Source: CAD feature listing. Evaluate the final solid. Frame: model axes, mm. A direction names the side the tool comes from. Coordinates: 2 decimals unless noted, no trailing zeros. Write each loop counter-clockwise with the first axis right and the second up, starting at its lowest first coordinate (ties: lowest second). Pieces come first, ordered by that corner, then holes. Notation, with made-up numbers: (34.5, -28) - (60.5, -28) arc R35 cw to (60.5, 11) - close; hole circle Ø9 at (16, 56). An arc over 180 degrees is marked (long way). One line per question, with ' | ' between items.
from build123d import *

# Parameters (mm, degrees)
CUT_EXTRUDE1_DEPTH      = 103.528044944
CUT_EXTRUDE1_DEPTH_BACK = 103.528044944
CUT_EXTRUDE2_DEPTH      = 104.553789555
CUT_EXTRUDE2_DEPTH_BACK = 104.553789555


with BuildPart() as part:
    # Sketch1 → Revolve1 (revolve)
    with BuildSketch(Plane.XY, mode=Mode.PRIVATE) as revolve1_sk:
        Polygon((0, 100), (-16, 10), (-16, 0), (0, 0), align=None)
    revolve(revolve1_sk.sketch.rotate(Axis((0, 0, 0), (0, 1, 0)), 270), axis=Axis((0, 0, 0), (0, 1, 0)))

    # Sketch3 → Cut-Extrude1 (cut, two sides: drawn at the far end of the back side and taken through both)
    with BuildSketch(Plane(origin=(0, 0, 0), x_dir=(0, 0, -1), z_dir=(1, 0, 0)).offset(-CUT_EXTRUDE1_DEPTH_BACK)):
        Polygon((-29.451982923, 10), (-6.451982923, 10), (-2.451982923, 110.819600833), (-29.451982923, 110.819600833), align=None)
        Polygon((29.451982923, 10), (6.451982923, 10), (2.451982923, 110.819600833), (29.451982923, 110.819600833), align=None)
    extrude(amount=CUT_EXTRUDE1_DEPTH + CUT_EXTRUDE1_DEPTH_BACK, mode=Mode.SUBTRACT)

    # Sketch4 → Cut-Extrude2 (cut, two sides: drawn at the far end of the back side and taken through both)
    with BuildSketch(Plane(origin=(0, 0.271295166, 6.837967583), x_dir=(1, 0, 0), z_dir=(0, 0.03964363571474905, 0.9992138820829684)).offset(-CUT_EXTRUDE2_DEPTH_BACK)):
        Polygon((-10, 9.73635876), (10, 9.73635876), (0, 93.839476738), align=None)
    extrude(amount=CUT_EXTRUDE2_DEPTH + CUT_EXTRUDE2_DEPTH_BACK, mode=Mode.SUBTRACT)


solid = part.part
Item 1: Mould query, pull axis Y, two halves, no side actions, for faces 4 (the face through (8.455, 32.54, 5.558)), 5 (the face through (-0.14, 9.55, -4.93)), 6 (the face through (0, 0, 0)). Classes: pulls with the +Y half, pulls with the -Y half, needs draft (parallel to the pull), parting line crosses it, or undercut.
Check sheet entries:
face 4: pulls with the +Y half | face 5: undercut | face 6: pulls with the -Y half
Item 2: Access query for faces 1 (the face through (0, 10, 10)), 2 (the face through (-0.703, 4.93, 15.985)), 3 (the face through (12, 10, -9)). Directions: +Z, -Z, +X, -X, +Y, -Y. A direction counts if a zero-diameter tool reaches every point of the face in a straight line with its end or side. Return the directions, or none.
Check sheet entries:
face 1: +Z, +X, -X, +Y | face 2: +Y, -Y | face 3: -Z, +X, -X, +Y
Item 3: Cut plane A-A on y = 11. Return loops of the section in (x, z), and give its area (3 significant figures).
Check sheet entries:
outline: (-14.46, -6.41) - (-9.82, -6.41) - (-9.88, 6.41) - (-14.46, 6.41) arc R15.82 ccw to start; (9.82, -6.41) - (14.46, -6.41) arc R15.82 ccw to (14.46, 6.41) - (9.88, 6.41) - close | area: 142 mm²
Item 4: Cut plane D-D on z = 9.5. Return loops of the section in (x, y), and give its area (3 significant figures).
Check sheet entries:
outline: (-12.87, 0) - (12.87, 0) - (12.87, 10) - (-12.87, 10) - close | area: 257 mm²
Item 5: Ray query, line 1 along X through (y, z) = (90.5, 1); line 2 along Z through (x, y) = (2.5, 74); line 3 along Y through (x, z) = (-2, 12). Return the intervals inside material, ascending. Write a range as [from, to].
Check sheet entries:
line 1: [-1.36, -0.41], [0.41, 1.36] | line 2: [-3.89, 3.89] | line 3: [0, 10]
Item 6: Cut plane C-C on y = 25.5. Return loops of the section in (x, z), and give its area (3 significant figures).
Check sheet entries:
outline: (-11.89, -5.84) - (-8.1, -5.84) - (-8.16, 5.84) - (-11.89, 5.84) arc R13.24 ccw to start; (8.1, -5.84) - (11.89, -5.84) arc R13.24 ccw to (11.89, 5.84) - (8.16, 5.84) - close | area: 109 mm²
Item 7: Pin query (flat end, axial travel): pin 1 Ø8 at (y, z) = (69, -4) entering from -X; pin 2 Ø10 at (x, y) = (2, 14) entering from -Z; pin 3 Ø5 at (y, z) = (50, -1.5) entering from +X. Return the tip coordinate at first contact, or that it passes through.
Check sheet entries:
pin 1: x = -5.9 | pin 2: z = -15.97 | pin 3: x = 9.28
Item 8: Cut plane B-B on z = -8. Return loops of the section in (x, y), and give its area (3 significant figures).
Check sheet entries:
outline: (-13.86, 0) - (13.86, 0) - (13.86, 10) - (9.93, 10) - (10, 9.43) - (-10, 9.43) - (-9.93, 10) - (-13.86, 10) - close | area: 266 mm²
